Read the model definition and answer for the solid it produces. Units are mm, in the model's axes. A direction names the side the tool comes from. Give positions to 0.01 mm unless a question says otherwise; leave off trailing zeros. Order: outer loops, then holes, each group sorted by start corner. A loop starts at its lowest first (then second) coordinate and runs counter-clockwise, first axis right, second up.
```python
from build123d import *

# Parameters (mm, degrees)
SKETCH1_W           = 170
SKETCH1_H           = 120
BOSS_EXTRUDE1_DEPTH = 7
SKETCH2_W           = 72
SKETCH2_H           = 26.620567464
CUT_EXTRUDE1_DEPTH  = 7
SKETCH3_R           = 2
CUT_EXTRUDE5_DEPTH  = 7
SKETCH7_R           = 2
CUT_EXTRUDE7_DEPTH  = 10
SKETCH6_R           = 2
CUT_EXTRUDE10_DEPTH = 10
SKETCH9_R           = 2
CUT_EXTRUDE11_DEPTH = 10
FILLET1_R           = 5


with BuildPart() as part:
    # Sketch1 → Boss-Extrude1 (new body)
    with BuildSketch(Plane(origin=(0, 0, 0), x_dir=(1, 0, 0), z_dir=(0, 1, 0))):
        Rectangle(SKETCH1_W, SKETCH1_H)
    extrude(amount=BOSS_EXTRUDE1_DEPTH)

    # Sketch2 → Cut-Extrude1 (cut)
    with BuildSketch(Plane(origin=(0, 7, 0), x_dir=(1, 0, 0), z_dir=(0, 1, 0))):
        with Locations((0, 1.926488435)):
            Rectangle(SKETCH2_W, SKETCH2_H)
    extrude(amount=-CUT_EXTRUDE1_DEPTH, mode=Mode.SUBTRACT)

    # Sketch3 → Cut-Extrude5 (cut)
    with BuildSketch(Plane(origin=(0, 7, 0), x_dir=(1, 0, 0), z_dir=(0, 1, 0))):
        with Locations((-80, 55)):
            Circle(SKETCH3_R)
    extrude(amount=-CUT_EXTRUDE5_DEPTH, mode=Mode.SUBTRACT)

    # Sketch7 → Cut-Extrude7 (cut)
    with BuildSketch(Plane(origin=(0, 7, 0), x_dir=(1, 0, 0), z_dir=(0, 1, 0))):
        with Locations((-80, -55)):
            Circle(SKETCH7_R)
    extrude(amount=-CUT_EXTRUDE7_DEPTH, mode=Mode.SUBTRACT)

    # Sketch6 → Cut-Extrude10 (cut)
    with BuildSketch(Plane(origin=(0, 7, 0), x_dir=(1, 0, 0), z_dir=(0, 1, 0))):
        with Locations((80, 55)):
            Circle(SKETCH6_R)
    extrude(amount=-CUT_EXTRUDE10_DEPTH, mode=Mode.SUBTRACT)

    # Sketch9 → Cut-Extrude11 (cut)
    with BuildSketch(Plane(origin=(0, 7, 0), x_dir=(1, 0, 0), z_dir=(0, 1, 0))):
        with Locations((80, -55)):
            Circle(SKETCH9_R)
    extrude(amount=-CUT_EXTRUDE11_DEPTH, mode=Mode.SUBTRACT)

    # Fillet1
    fillet1_edges = [part.edges().sort_by_distance(p)[0] for p in [
        (-85, 3.5, -60),
        (85, 3.5, -60),
        (85, 3.5, 60),
        (-85, 3.5, 60),
    ]]
    fillet(fillet1_edges, radius=FILLET1_R)


solid = part.part
```
1) For a pull along X with two mould halves and no side action, classify faces 3 (the face through (-36, 4, -2)), 4 (the face through (-1, 4, -15.237)), 5 (the face through (-85, 3, 1)), 6 (the face through (-1, 3, 60)) as released by +X, released by -X, zero draft, split by the parting line, or undercut.
Final values:
face 3: undercut
face 4: undercut
face 5: released by -X
face 6: zero draft
2) Consider L1, parallel to Z at x = 80, y = 5.75; L2, parallel to X at y = 5.75, z = 55; L3, parallel to Z at x = -17, y = 2.5. Determine where each line is inside the solid, lowest interval first.
Final values:
L1: z = -60 to -57, -53 to 53, 57 to 60
L2: x = -85 to -82, -78 to 78, 82 to 85
L3: z = -60 to -15.24, 11.38 to 60
3) Given pin 1 (5 mm diameter, centred on x = -80, z = -55, fed in from +Y), flat-ended and moving along its own axis, determine where the tip first touches the part or whether it passes through.
Final values:
pin 1: stops at y = 7
4) A tool of negligible diameter and unlimited length cuts with its end or side. For faces 1 (the face through (85, 3, 1)), 2 (the face through (-1, 4, 11.384)), from which of +Z, -Z, +X, -X, +Y, -Y can it reach the whole face along a straight path? Write none if from no direction.
Final values:
face 1: +Z, -Z, +X, +Y, -Y
face 2: +Y, -Y
5) The part is cut by section C-C on y = 4.5. Determine the outline of the cut face in (x, z), and give its area (3 significant figures).
Final values:
outline: (-85, -55) arc R5 ccw to (-80, -60) - (80, -60) arc R5 ccw to (85, -55) - (85, 55) arc R5 ccw to (80, 60) - (-80, 60) arc R5 ccw to (-85, 55) - close; hole circle Ø4 at (-80, -55); hole circle Ø4 at (-80, 55); hole (-36, -15.24) - (36, -15.24) - (36, 11.38) - (-36, 11.38) - close; hole circle Ø4 at (80, -55); hole circle Ø4 at (80, 55)
area: 18,400 mm2
6) The part is cut by section B-B on z = -3.5. Determine the outline of the cut face in (x, y), and give its area (3 significant figures).
Final values:
outline: (-85, 0) - (-36, 0) - (-36, 7) - (-85, 7) - close; (36, 0) - (85, 0) - (85, 7) - (36, 7) - close
area: 686 mm2
7) The part is cut by section A-A on x = 4. Determine the outline of the cut face in (y, z).
Final values:
outline: (0, -60) - (7, -60) - (7, -15.24) - (0, -15.24) - close; (0, 11.38) - (7, 11.38) - (7, 60) - (0, 60) - close
